from build123d import *

# Parameters (mm, degrees)
SKETCH_1_R      = 59
SKETCH_1_R_2    = 51.5
SKETCH_1_R_3    = 1.6
EXTRUDE_1_DEPTH = 3


with BuildPart() as part:
    # 草图1 → 凸台-拉伸1 (new body)
    with BuildSketch(Plane.XY):
        Circle(SKETCH_1_R)
        Circle(SKETCH_1_R_2, mode=Mode.SUBTRACT)
        with Locations((16.5, 51.942275653)):
            Circle(SKETCH_1_R_3, mode=Mode.SUBTRACT)
        with Locations((22.5, 49.638694584)):
            Circle(SKETCH_1_R_3, mode=Mode.SUBTRACT)
        with Locations((53.047148839, 12.5)):
            Circle(SKETCH_1_R_3, mode=Mode.SUBTRACT)
        with Locations(Location((22.5, -49.638694584, 0), (0, 0, 180))):
            Circle(SKETCH_1_R_3, mode=Mode.SUBTRACT)
        with Locations(Location((16.5, -51.942275653, 0), (0, 0, 180))):
            Circle(SKETCH_1_R_3, mode=Mode.SUBTRACT)
        with Locations(Location((53.047148839, -12.5, 0), (0, 0, 180))):
            Circle(SKETCH_1_R_3, mode=Mode.SUBTRACT)
        with Locations((-16.5, -51.942275653)):
            Circle(SKETCH_1_R_3, mode=Mode.SUBTRACT)
        with Locations((-22.5, -49.638694584)):
            Circle(SKETCH_1_R_3, mode=Mode.SUBTRACT)
        with Locations((-53.047148839, -12.5)):
            Circle(SKETCH_1_R_3, mode=Mode.SUBTRACT)
        with Locations(Location((-53.047148839, 12.5, 0), (0, 0, 180))):
            Circle(SKETCH_1_R_3, mode=Mode.SUBTRACT)
        with Locations(Location((-22.5, 49.638694584, 0), (0, 0, 180))):
            Circle(SKETCH_1_R_3, mode=Mode.SUBTRACT)
        with Locations(Location((-16.5, 51.942275653, 0), (0, 0, 180))):
            Circle(SKETCH_1_R_3, mode=Mode.SUBTRACT)
    extrude(amount=EXTRUDE_1_DEPTH)


solid = part.part
The listing builds one solid part. Answer for the finished solid, in the listing's coordinates (mm). Round coordinates to 2 decimals unless told otherwise and drop trailing zeros. Order: outer loops, then holes, each group sorted by start corner. A loop starts at its lowest first (then second) coordinate and runs counter-clockwise, first axis right, second up. Notation, with made-up numbers: M 30.5,-39 L 79.5,-39 A23 ccw 79.5,-9 Z; hole C 82.25,-17 d4. An arc over 180 degrees is marked long. Answer in a Markdown table with one row per item. Add a question column.
1) Flat-ended cylindrical pins translate along their axes: pin 1 Ø5 at (x, y) = (41, -33) entering from -Z; pin 2 Ø2.5 at (x, y) = (-53.05, -12.5) entering from +Z. Find the tip coordinate at first contact, or state that the pin passes through.
2) Consider line 1 along Y through (x, z) = (-23.5, 2.8); line 2 along Y through (x, z) = (16.5, 0.75); line 3 along Y through (x, z) = (-52.5, 2.5). Determine where each line is inside the solid, lowest interval first. Write a range as from..to.
3) Determine the mould class of faces 1 (the face through (-14.9, 51.9, 1.5)), 2 (the face through (0, -52, 3)), 3 (the face through (56.275, 17.722, 1.479)) for opening direction Y: pulls with the +Y half, pulls with the -Y half, needs draft (parallel to the pull), parting line crosses it, or undercut.
4) The part is cut by section D-D on z = 2.3. Count the separate pieces of the cut face and the enclosed holes in it, plus the area to 3 significant figures.
5) The part is cut by section C-C on x = -16.5. Determine the outline of the cut face in (y, z).
6) The part is cut by section A-A on y = 0. Determine the outline of the cut face in (x, z), plus the area to 3 significant figures.
Findings below:
| question | item | result |
|---|---|---|
| 1 | pin 1 | stops at z = 0 |
| 1 | pin 2 | passes through |
| 2 | line 1 | y = -54.12..-50.89, -48.39..-45.83, 45.83..48.39, 50.89..54.12 |
| 2 | line 2 | y = -56.65..-53.54, -50.34..-48.79, 48.79..50.34, 53.54..56.65 |
| 2 | line 3 | y = -26.92..-14, -11..11, 14..26.92 |
| 3 | face 1 | undercut |
| 3 | face 2 | needs draft |
| 3 | face 3 | parting line crosses it |
| 4 | separate pieces | 1 |
| 4 | enclosed holes | 13 |
| 4 | area | 2,510 mm² |
| 5 | outline | M -56.65,0 L -53.54,0 L -53.54,3 L -56.65,3 Z; M -50.34,0 L -48.79,0 L -48.79,3 L -50.34,3 Z; M 48.79,0 L 50.34,0 L 50.34,3 L 48.79,3 Z; M 53.54,0 L 56.65,0 L 56.65,3 L 53.54,3 Z |
| 6 | outline | M -59,0 L -51.5,0 L -51.5,3 L -59,3 Z; M 51.5,0 L 59,0 L 59,3 L 51.5,3 Z |
| 6 | area | 45.0 mm² |
